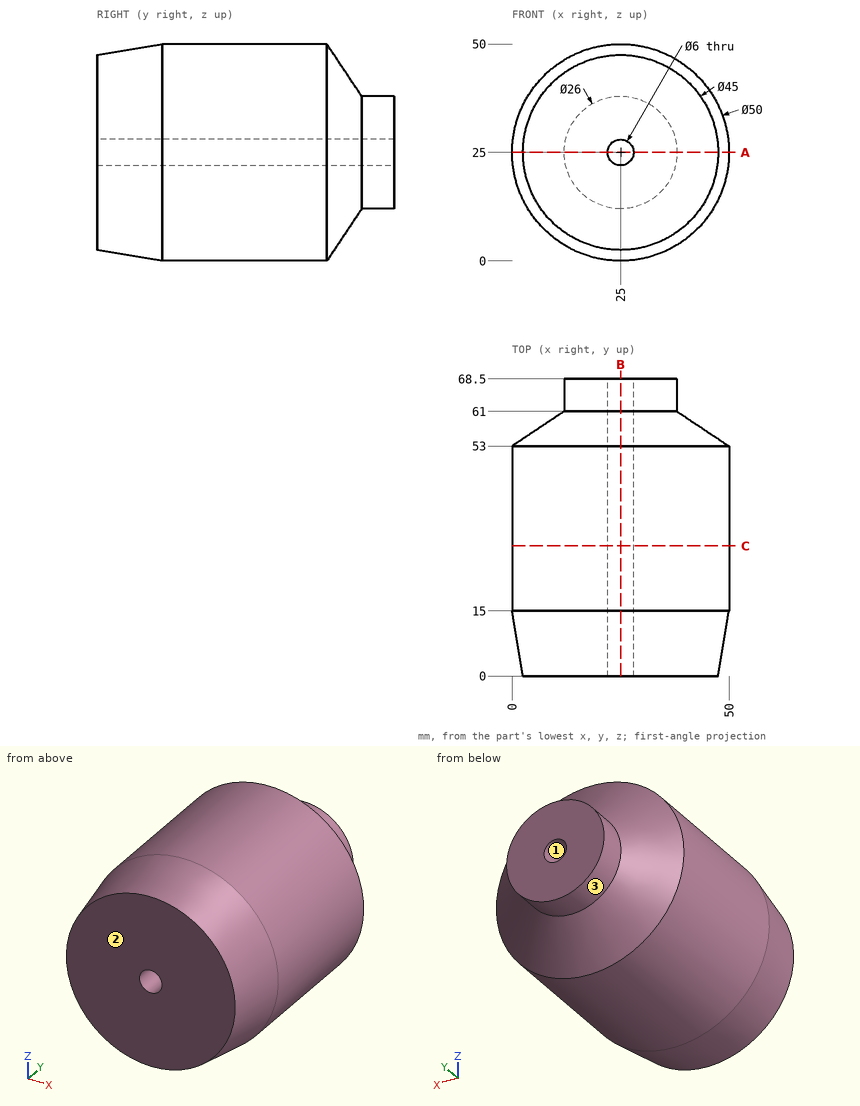
Here's the drawing with two shaded views (mm, measured from the low corner). I have some questions. Round coordinates to 2 decimals unless told otherwise and drop trailing zeros. Loops run counter-clockwise (first coordinate to the right, second up) from the corner with the lowest first, then second, coordinate; pieces in that order, holes last. Notation, with made-up numbers: M 12,27 L 32,27 A16 ccw 32,56 Z; hole C 62.5,15 d6. An arc over 180 degrees is marked long. Put each result on its own line as item: value.
Q1. I need wall thicknesses on probe 1 along X at (y, z) = (48.5, 25); probe 2 along X at (y, z) = (7.5, 22.5); probe 3 along Z at (x, y) = (24, 48.5). Which ranges of each line are inside material? Lowest first, please.
Check result:
probe 1: 0 to 22, 28 to 50
probe 2: 1.38 to 23.34, 26.66 to 48.62
probe 3: 0.02 to 22.17, 27.83 to 49.98
Q2. Imagine slicing it at C-C (y = 30). Write out the boundary of the cut face in (x, z).
Check result:
outline: C 25,25 d50; hole C 25,25 d6
Q3. Imagine slicing it at A-A (z = 25). Write out the boundary of the cut face in (x, y), then the cut area to 3 significant figures.
Check result:
outline: M 0,15 L 2.5,0 L 22,0 L 22,68.5 L 12,68.5 L 12,61 L 0,53 Z; M 28,0 L 47.5,0 L 50,15 L 50,53 L 38,61 L 38,68.5 L 28,68.5 Z
area: 2,700 mm2
Q4. Thinking about a two-plate mould opening in X: for the marked faces 1, 2 and 3, which applies, released by +X, released by -X, zero draft, split by the parting line, or undercut?
Check result:
face 1: undercut
face 2: zero draft
face 3: split by the parting line
Q5. For pin 1 (2 mm diameter, centred on y = 58.5, z = 24, fed in from -X); pin 2 (5 mm diameter, centred on y = 11.5, z = 25.5, fed in from -X); pin 3 (3 mm diameter, centred on x = 21, y = 59.5, fed in from +Z), each with a flat end and sliding along its axis, tell me the tip position at first contact or that it passes through.
Check result:
pin 1: x = 6.78
pin 2: x = 0.17
pin 3: z = 42.06
Q6. Imagine slicing it at B-B (x = 25). Write out the boundary of the cut face in (y, z).
Check result:
outline: M 0,2.5 L 15,0 L 53,0 L 61,12 L 68.5,12 L 68.5,22 L 0,22 Z; M 0,28 L 68.5,28 L 68.5,38 L 61,38 L 53,50 L 15,50 L 0,47.5 Z
